Autodesk Inventor part; units mm, degrees
ref_plane "YZ Plane" through (0, 0, 0) normal (1, 0, 0) x (0, 1, 0)
ref_plane "XZ Plane" through (0, 0, 0) normal (0, 1, 0) x (-1, 0, 0)
ref_plane "XY Plane" through (0, 0, 0) normal (0, 0, 1) x (1, 0, 0)
sketch "Эскиз1" plane through (0, 0, 0) normal (1, 0, 0) x (0, 1, 0)
  line L0 (0, 0) -> (143.27187, 0) construction
  line L1 (0, 0) -> (0, -170.504512) construction
  arc A0 (0, -8.91) -> (-8.91, 0) centre (0, 0) ccw
  circle A1 centre (0, -52.3) radius 7.5
  circle A2 centre (0, 0) radius 7.5
  line L2 (-8.91, 0) -> (-8.91, -52.3)
  line L3 (-5.91, -10.91) -> (-5.91, -41.39)
  line L4 (0, -8.91) -> (-3.91, -8.91)
  line L5 (0, -43.39) -> (-3.91, -43.39)
  line L6 (-12.45, -60.45) -> (-12.45, -57.11)
  line L7 (-12.45, -57.11) -> (-11.45, -57.11)
  line L8 (-11.45, -57.11) -> (-11.45, -59.11)
  line L9 (-11.45, -59.11) -> (-8.0282, -59.11)
  arc A3 (-8.91, -52.3) -> (-7.218089, -57.523724) centre (0, -52.3) ccw
  arc A4 (-3.267299, -60.589322) -> (0, -43.39) centre (0, -52.3) ccw
  circle A5 centre (0, 0) radius 4 construction
  line L10 (0, 4) -> (-17.853128, 4) construction
  line L11 (-17.853128, 4) -> (-17.853128, -60.45) construction
  line L12 (-17.853128, -60.45) -> (-12.45, -60.45) construction
  line L13 (-12.45, -60.45) -> (-4.0007, -60.45)
  arc A6 (-8.0282, -59.11) -> (-7.218089, -57.523724) centre (-8.0282, -58.11) ccw
  arc A7 (-5.91, -41.39) -> (-3.91, -43.39) centre (-3.91, -41.39) ccw
  arc A8 (-3.91, -8.91) -> (-5.91, -10.91) centre (-3.91, -10.91) ccw
  arc A9 (-3.267299, -60.589322) -> (-4.0007, -60.45) centre (-4.0007, -62.45) ccw
  point P0 (-5.91, -43.39)
  point P1 (-5.91, -8.91)
  point P2 (0, -61.21)
  point P3 (-5.745607, -59.11)
  point P4 (-3.600778, -60.45)
  dimension "d34" = 8
  dimension "d0" = 17.82
  dimension "d2" = 15
  dimension "d3" = 15
  dimension "d4" = 52.3
  dimension "d5" = 3
  dimension "d9" = 1
  dimension "d11" = 8.91
  dimension "d12" = 8.91
  dimension "d13" = 3.54
  dimension "d35" = 64.45
  dimension "d36" = 3.34
  dimension "d37" = 1.34
  dimension "d38" = 1
  dimension "d39" = 2
  dimension "d40" = 2
  dimension "d41" = 2
  dimension "d42" = 63.11
  dimension "d43" = 70.12
extrude "Выдавливание1" add sketch "Эскиз1" along normal mid plane 50
sketch "Эскиз2" plane through (-25, -5.91, -8.91) normal (0, 1, 0) x (1, 0, 0)
  circle A0 centre (13.95, 28.46) radius 5.95
  line L0 (4.95, 28.46) -> (13.95, 28.46) construction
  line L1 (13.95, 28.46) -> (24.436318, 28.46) construction
  circle A1 centre (4.95, 28.46) radius 1.6
  circle A2 centre (22.95, 28.46) radius 1.6
  line L2 (13.95, 28.46) -> (13.95, 32.27883)
  circle A3 centre (4.95, 28.46) radius 1.455 construction
  circle A4 centre (22.95, 28.46) radius 1.455 construction
  line L3 (0, 5.642815) -> (0, 38.122815) construction
  line L4 (50, -8.91) -> (50, 43.39) construction
  line L5 (50, 14.93) -> (39.51, 14.93)
  line L6 (39.51, 14.93) -> (39.51, 33.09)
  line L7 (39.51, 33.09) -> (50, 33.09)
  line L8 (50, 33.09) -> (50, 14.93)
  line L9 (0, -18.82) -> (50, -18.82) construction
  line L10 (50, 43.39) -> (2.383382, 43.39)
  line L11 (50, -17.82) -> (50, 0)
  line L12 (50, -17.82) -> (50, 0)
  line L13 (50, -8.91) -> (53.294914, -8.91)
  line L14 (50, -12.91) -> (54.162489, -12.91)
  line L15 (0, 52.3) -> (50, 52.3)
  dimension "d15" = 3.2
  dimension "d16" = 3.2
  dimension "d17" = 2.91
  dimension "d18" = 2.91
  dimension "d21" = 18
  dimension "d22" = 11.9
  dimension "d23" = 8
  dimension "d25" = 39.51
  dimension "d27" = 18.16
  dimension "d44" = 17.82
  dimension "d45" = 8.91
  dimension "d46" = 8.91
  dimension "d48" = 4
  dimension "d49" = 46
  dimension "d50" = 10.49
  dimension "d51" = 19.61
  dimension "d52" = 17.89
extrude "Выдавливание2" cut sketch "Эскиз2" along normal mid plane 50
sketch "Эскиз4" plane through (-25, -5.91, -10.91) normal (0, 1, 0) x (1, 0, 0)
  line L0 (14.05, 0.23) -> (37.55, 0.23) construction
  circle A0 centre (14.05, 0.23) radius 2.05
  circle A1 centre (37.55, 0.23) radius 2.05
  line L1 (0, -19.82) -> (50, -19.82) construction
  line L2 (0, 0) -> (0, 30.48) construction
  line L3 (50, 12.93) -> (50, 0)
  point P0 (25, -10.91)
  dimension "d53" = 4.1
  dimension "d54" = 4.1
  dimension "d57" = 18
  dimension "d61" = 19.4
  dimension "d63" = 14.05
  dimension "d65" = 23.5
extrude "Выдавливание3" cut sketch "Эскиз4" along normal mid plane 50
sketch "Эскиз6" plane through (-25, -5.91, -10.91) normal (0, 1, 0) x (1, 0, 0)
  circle A0 centre (42, 7.46) radius 1.5
  arc A1 (16.087057, 0) -> (12.012943, 0) centre (14.05, 0.23) ccw
  circle A2 centre (14.05, 0.23) radius 2
  arc A3 (39.587057, 0) -> (35.512943, 0) centre (37.55, 0.23) ccw
  circle A4 centre (37.55, 0.23) radius 2
  circle A5 centre (24, 7.46) radius 1.5
  circle A6 centre (4.95, 26.46) radius 1.129269
  spline S0 degree 3 poles (21.799899, 26.563204) (21.753431, 26.045363) (22.103055, 25.518519) (22.59827, 25.36015) (23.093485, 25.201782) (23.683934, 25.427991) (23.946568, 25.876703) (24.209201, 26.325414) (24.117313, 26.951) (23.73674, 27.305235) (23.356167, 27.659471) (22.725608, 27.706335) (22.296851, 27.41225) (21.868094, 27.118165) (21.684738, 26.513036) (21.878155, 26.03043) (22.071571, 25.547824) (22.622094, 25.236816) (23.135279, 25.320239) (23.648464, 25.403662) (24.072128, 25.873034) (24.102721, 26.392055) (24.133314, 26.911075) (23.767725, 27.426968) (23.267894, 27.570102) (22.768063, 27.713236) (22.184816, 27.469056) (21.936042, 27.012515) (21.687268, 26.555973) (21.798265, 25.933494) (22.189505, 25.591075) (22.580744, 25.248657) (23.212442, 25.221119) (23.631995, 25.528192) (24.051548, 25.835265) (24.216293, 26.445724) (24.008192, 26.922183) (23.800091, 27.398641) (23.240306, 27.692649) (22.729915, 27.593554) (22.219524, 27.494459) (21.810428, 27.012338) (21.795739, 26.492624) (21.78105, 25.972909) (22.162261, 25.468451) (22.66624, 25.340686) (23.170219, 25.212921) (23.745717, 25.474842) (23.980398, 25.938786) (24.215078, 26.40273) (24.085076, 27.021519) (23.683537, 27.3518) (23.281998, 27.68208) (22.649753, 27.690266) (22.239798, 27.370492) (21.829842, 27.050718) (21.683864, 26.435502) (21.906453, 25.965638) (22.129043, 25.495774) (22.697567, 25.219041) (23.204685, 25.333715) (23.711803, 25.448389) (24.105947, 25.942808) (24.104719, 26.462729) (24.10349, 26.982649) (23.707014, 27.475201) (23.199359, 27.587476) (22.691705, 27.699752) (22.124496, 27.420335) (21.904129, 26.949424) (21.683762, 26.478514) (21.832647, 25.863994) (22.244109, 25.546162) (22.655571, 25.228329) (23.28777, 25.239503) (23.687744, 25.571677) (24.087717, 25.903851) (24.214793, 26.523248) (23.977923, 26.986078) (23.741053, 27.448907) (23.164323, 27.708105) (22.660954, 27.57796) (22.157584, 27.447815) (21.778761, 26.94156) (21.795906, 26.421922) (21.813051, 25.902283) (22.224421, 25.4221) (22.735274, 25.325418) (23.246128, 25.228736) (23.804518, 25.525387) (24.010365, 26.002824) (24.216211, 26.48026) (24.048583, 27.089934) (23.627584, 27.39502) (23.206584, 27.700107) (22.575023, 27.669584) (22.185407, 27.325321) (21.79579, 26.981057) (21.687736, 26.35806) (21.938665, 25.9027) (22.189593, 25.447339) (22.773988, 25.205918) (23.273137, 25.351413) (23.772286, 25.496907) (24.135433, 26.014522) (24.102387, 26.533393) (24.069342, 27.052263) (23.643464, 27.519627) (23.12989, 27.600624) (22.616316, 27.681621) (22.06727, 27.368014) (21.876136, 26.8845) (21.685002, 26.400985) (21.871217, 25.796729) (22.301359, 25.504674) (22.731501, 25.212619) (23.361832, 25.262462) (23.740726, 25.618492) (24.119621, 25.974522) (24.208551, 26.600535) (23.9438, 27.048001) (23.679048, 27.495466) (23.087537, 27.718883) (22.593076, 27.558175) (22.098615, 27.397467) (21.751485, 26.868978) (21.8004, 26.351362) (21.849315, 25.833747) (22.289301, 25.37964) (22.805114, 25.314404) (23.320926, 25.249168) (23.860114, 25.579436) (24.036356, 26.068575) (24.212598, 26.557715) (24.007972, 27.155986) (23.56909, 27.434736) (23.130209, 27.713486) (22.5017, 27.644368) (22.133882, 27.276906) (21.961347, 27.104537) (21.845629, 26.876206) (21.808638, 26.635144) knots 2.61665571 2.61665571 2.61665571 2.61665571 3.96742673 3.96742673 3.96742673 5.31819776 5.31819776 5.31819776 6.66896878 6.66896878 6.66896878 8.01973981 8.01973981 8.01973981 9.37051084 9.37051084 9.37051084 10.72128186 10.72128186 10.72128186 12.07205289 12.07205289 12.07205289 13.42282392 13.42282392 13.42282392 14.77359494 14.77359494 14.77359494 16.12436597 16.12436597 16.12436597 17.475137 17.475137 17.475137 18.82590802 18.82590802 18.82590802 20.17667905 20.17667905 20.17667905 21.52745007 21.52745007 21.52745007 22.8782211 22.8782211 22.8782211 24.22899213 24.22899213 24.22899213 25.57976315 25.57976315 25.57976315 26.93053418 26.93053418 26.93053418 28.28130521 28.28130521 28.28130521 29.63207623 29.63207623 29.63207623 30.98284726 30.98284726 30.98284726 32.33361829 32.33361829 32.33361829 33.68438931 33.68438931 33.68438931 35.03516034 35.03516034 35.03516034 36.38593137 36.38593137 36.38593137 37.73670239 37.73670239 37.73670239 39.08747342 39.08747342 39.08747342 40.43824444 40.43824444 40.43824444 41.78901547 41.78901547 41.78901547 43.1397865 43.1397865 43.1397865 44.49055752 44.49055752 44.49055752 45.84132855 45.84132855 45.84132855 47.19209958 47.19209958 47.19209958 48.5428706 48.5428706 48.5428706 49.89364163 49.89364163 49.89364163 51.24441266 51.24441266 51.24441266 52.59518368 52.59518368 52.59518368 53.94595471 53.94595471 53.94595471 55.29672574 55.29672574 55.29672574 56.64749676 56.64749676 56.64749676 57.99826779 57.99826779 57.99826779 59.34903881 59.34903881 59.34903881 60.69980984 60.69980984 60.69980984 62.05058087 62.05058087 62.05058087 63.40135189 63.40135189 63.40135189 64.75212292 64.75212292 64.75212292 65.38573969 65.38573969 65.38573969 65.38573969
  circle A7 centre (22.95, 26.46) radius 1.6
  circle A8 centre (22.95, 26.46) radius 1.154622
  circle A9 centre (4.95, 26.46) radius 2.474109
  line L0 (-39.849119, 12.49) -> (304.043155, 12.49)
  line L1 (39.51, 31.09) -> (50, 31.09)
  line L2 (39.51, 12.93) -> (39.51, 30.48)
  line L3 (50, 12.93) -> (50, 0)
  point P0 (25, -10.91)
  dimension "d66" = 3
  dimension "d67" = 4
  dimension "d68" = 4
  dimension "d70" = 3
  dimension "d72" = 19
  dimension "d73" = 19
  dimension "d74" = 12.26
  dimension "d75" = 30.86
  dimension "d76" = 23.63
  dimension "d78" = 8
  dimension "d79" = 18
extrude "Выдавливание4" cut sketch "Эскиз6" against normal blind 10 contours A0 | A5
properties part number "каретка  хотэнда"
Verification items for the finished model (mm, model axes). A direction names the side the tool comes from. Give positions to 0.01 mm unless a question says otherwise; leave off trailing zeros. Loops run counter-clockwise (first coordinate to the right, second up) from the corner with the lowest first, then second, coordinate; pieces in that order, holes last. Notation, with made-up numbers: M 24,8.25 L 58,8.25 A30 cw 58,45.25 Z; hole C 7,70 d10. An arc over 180 degrees is marked long. Return JSON: item names as keys, results as strings.
1) Section check B-B, the plane z = -37.37. Enter the section's corners in (x, y), and give its area (3 significant figures).
Findings:
{"outline": "M -25,-8.91 L -21.65,-8.91 L -21.65,-5.91 L -25,-5.91 Z; M -18.45,-8.91 L -17,-8.91 L -17,-5.91 L -18.45,-5.91 Z; M -5.1,-8.91 L -3.65,-8.91 L -3.65,-5.91 L -5.1,-5.91 Z; M -0.45,-8.91 L 14.51,-8.91 L 14.51,-5.91 L -0.45,-5.91 Z", "area": "63.6 mm2"}
2) Section check D-D, the plane z = -46. Enter the section's corners in (x, y), and give its area (3 significant figures).
Findings:
{"outline": "M -25,-8.91 L 25,-8.91 L 25,-4.07 L -25,-4.07 Z; M -25,4.07 L 25,4.07 L 25,6.3 L -25,6.3 Z", "area": "354 mm2"}
3) Gauge pin test, flat ends, axial feed: P1, Ø2, axis at x = -10, z = -58.5, coming from the +Y side; P2, Ø6.5, axis at x = 12.55, z = -11.14, coming from the +Y side; P3, Ø5, axis at x = -20.05, z = -37.37, coming from the -Y side. Record the tip position at first contact, or that the pin passes through.
Findings:
{"P1": "stops at y = 7.24", "P2": "stops at y = 4.14", "P3": "stops at y = -8.91"}
4) Section check A-A, the plane x = 17. Enter the section's corners in (y, z).
Findings:
{"outline": "M -12.45,-60.45 L -4,-60.45 A2 cw -3.27,-60.59 A8.91 ccw long 0,-43.39 L -3.91,-43.39 A2 cw -5.81,-42 L -8.91,-42 L -8.91,-52.3 A8.91 ccw -7.22,-57.52 A1 cw -8.03,-59.11 L -11.45,-59.11 L -11.45,-57.11 L -12.45,-57.11 Z; M -8.91,-23.84 L -5.91,-23.84 L -5.91,-19.87 L -8.91,-19.87 Z; M -8.91,-16.87 L -5.91,-16.87 L -5.91,-10.91 A2 cw -3.91,-8.91 L 0,-8.91 A8.91 ccw long -8.91,0 Z; hole C 0,-52.3 d15; hole C 0,0 d15"}
5) Mould release check, pull along Z, two halves, no side actions. Record for faces 4 (the flat face through (0, -12.45, -59)), 5 (the flat face through (0, -8, -60.45)), 6 (the flat face through (0, -2, -8.91)): released by +Z, released by -Z, zero draft, split by the parting line, or undercut.
Findings:
{"face 4": "zero draft", "face 5": "released by -Z", "face 6": "undercut"}
6) Material ranges on L1, parallel to X at y = -6.7, z = -18.37; L2, parallel to X at y = -7, z = -11.14; L3, parallel to Z at x = 0, y = -0.5, recorded low to high. Write a range as [from, to].
Findings:
{"L1": "x = [-25, -2.5], [0.5, 15.5], [18.5, 25]", "L2": "x = [-25, -13], [-8.9, 10.5], [14.6, 25]", "L3": "z = [-61.2, -59.78], [-44.82, -43.39], [-8.91, -7.48], [7.48, 8.9]"}
7) Section check C-C, the plane x = -20.05. Enter the section's corners in (y, z), and give its area (3 significant figures).
Findings:
{"outline": "M -12.45,-60.45 L -4,-60.45 A2 cw -3.27,-60.59 A8.91 ccw long 0,-43.39 L -3.91,-43.39 A2 cw -5.91,-41.39 L -5.91,-38.97 L -8.91,-38.97 L -8.91,-52.3 A8.91 ccw -7.22,-57.52 A1 cw -8.03,-59.11 L -11.45,-59.11 L -11.45,-57.11 L -12.45,-57.11 Z; M -8.91,-35.77 L -5.91,-35.77 L -5.91,-10.91 A2 cw -3.91,-8.91 L 0,-8.91 A8.91 ccw long -8.91,0 Z; hole C 0,-52.3 d15; hole C 0,0 d15", "area": "288 mm2"}
8) Tool access check on faces 1 (the flat face through (20, -7, -23.84)), 2 (the flat face through (0, -10, -59.11)), 3 (the flat face through (0, -2, -43.39)). Record the directions out of +Z, -Z, +X, -X, +Y, -Y that give a thin tool (end or side, any length) a straight path to the whole face; none if there is none.
Findings:
{"face 1": "+X, +Y, -Y", "face 2": "+X, -X", "face 3": "+X, -X, +Y"}
